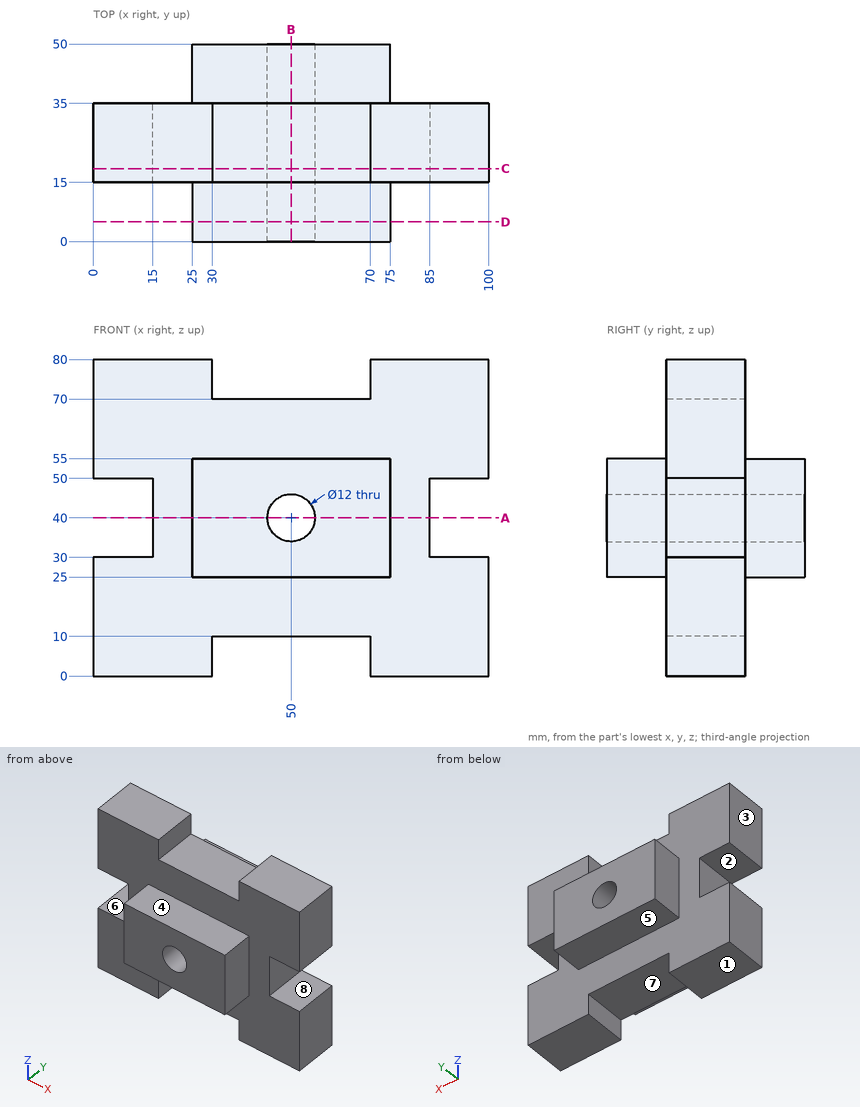
Drawing for the job (mm, zero at the part's lowest x, y, z). A direction names the side the tool comes from. Round coordinates to 2 decimals unless told otherwise and drop trailing zeros. Order: outer loops, then holes, each group sorted by start corner. A loop starts at its lowest first (then second) coordinate and runs counter-clockwise, first axis right, second up.
Item 1: Saw through at A-A on z = 40. Write the cut outline in (x, y), then the cut area to 3 significant figures.
Item 2: Pin check, flat tips, straight feed: pin 1 (4 mm diameter, centred on y = 11.5, z = 35.5, fed in from +X); pin 2 (22 mm diameter, centred on y = 22, z = 40.5, fed in from +X); pin 3 (1.5 mm diameter, centred on x = 81.5, z = 61, fed in from -Y); pin 4 (7.5 mm diameter, centred on x = 56, y = 7.5, fed in from -Z). Stop position of each tip, or through.
Item 3: Saw through at C-C on y = 18.5. Write the cut outline in (x, z).
Item 4: Tool access for the marked faces 4, 5, 6, 7 and 8: list every direction of +Z, -Z, +X, -X, +Y, -Y with a clear straight run to the whole face (end or side of a thin tool).
Item 5: Mould opens along Z. For the marked faces 1, 2 and 3 say: pulls with the +Z half, pulls with the -Z half, needs draft (parallel to the pull), parting line crosses it, or undercut.
Item 6: Saw through at B-B on x = 50. Write the cut outline in (y, z), then the cut area to 3 significant figures.
Item 7: Saw through at D-D on y = 5. Write the cut outline in (x, z), then the cut area to 3 significant figures.
Item 8: Probe line 1 along Z through (x, y) = (50, 22); line 2 along X through (y, z) = (30, 40); line 3 along X through (y, z) = (10, 40). List the from-to ranges inside material, lowest first.
Reported:
1. outline: (15, 15) - (25, 15) - (25, 0) - (44, 0) - (44, 50) - (25, 50) - (25, 35) - (15, 35) - close; (56, 0) - (75, 0) - (75, 15) - (85, 15) - (85, 35) - (75, 35) - (75, 50) - (56, 50) - close
1. area: 2,300 mm2
2. pin 1: stops at x = 75
2. pin 2: stops at x = 100
2. pin 3: stops at y = 15
2. pin 4: stops at z = 25
3. outline: (0, 0) - (30, 0) - (30, 10) - (70, 10) - (70, 0) - (100, 0) - (100, 30) - (85, 30) - (85, 50) - (100, 50) - (100, 80) - (70, 80) - (70, 70) - (30, 70) - (30, 80) - (0, 80) - (0, 50) - (15, 50) - (15, 30) - (0, 30) - close; hole circle Ø12 at (50, 40)
4. face 4: +Z, +X, -X, -Y
4. face 5: -Z, +X, -X, +Y
4. face 6: -X, +Y, -Y
4. face 7: -Z, +Y, -Y
4. face 8: +X, +Y, -Y
5. face 1: pulls with the -Z half
5. face 2: undercut
5. face 3: needs draft
6. outline: (0, 25) - (15, 25) - (15, 10) - (35, 10) - (35, 25) - (50, 25) - (50, 34) - (0, 34) - close; (0, 46) - (50, 46) - (50, 55) - (35, 55) - (35, 70) - (15, 70) - (15, 55) - (0, 55) - close
6. area: 1,500 mm2
7. outline: (25, 25) - (75, 25) - (75, 55) - (25, 55) - close; hole circle Ø12 at (50, 40)
7. area: 1,390 mm2
8. line 1: z = 10 to 34, 46 to 70
8. line 2: x = 15 to 44, 56 to 85
8. line 3: x = 25 to 44, 56 to 75
